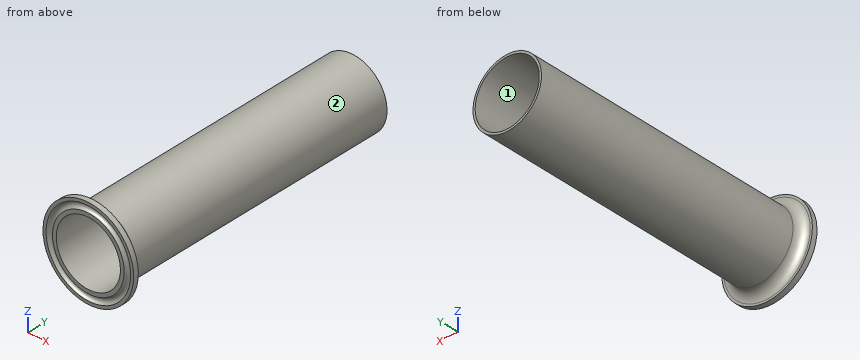
from build123d import *

# Parameters (mm, degrees)
SKETCH_1_R          = 25.25
EXTRUDE_1_DEPTH     = 2.8
SKETCH_2_R          = 19.05
EXTRUDE_2_DEPTH     = 157.2
FILLET_1_R          = 5
SKETCH_3_R          = 17.85
CUT_EXTRUDE_1_DEPTH = 164.936344354
SKETCH_5_R          = 1.8


with BuildPart() as part:
    # 스케치1 → 보스-돌출1 (new body)
    with BuildSketch(Plane(origin=(0, 0, 0), x_dir=(1, 0, 0), z_dir=(0, 1, 0))):
        with Locations(Location((0, 0, 0), (0, 0, 270))):
            Circle(SKETCH_1_R)
    extrude(amount=EXTRUDE_1_DEPTH)

    # 스케치2 → 보스-돌출2 (add)
    with BuildSketch(Plane(origin=(0, 2.8, 0), x_dir=(1, 0, 0), z_dir=(0, 1, 0))):
        with Locations(Location((0, 0, 0), (0, 0, 270))):
            Circle(SKETCH_2_R)
    extrude(amount=EXTRUDE_2_DEPTH)

    # 필렛1
    fillet_1_edges = [part.edges().sort_by_distance(p)[0] for p in [
        (0, 2.8, -19.05),
    ]]
    fillet(fillet_1_edges, radius=FILLET_1_R)

    # 스케치3 → 컷-돌출1 (cut, through all)
    with BuildSketch(Plane(origin=(0, 160, 0), x_dir=(1, 0, 0), z_dir=(0, 1, 0))):
        with Locations(Location((0, 0, 0), (0, 0, 270))):
            Circle(SKETCH_3_R)
    extrude(amount=-CUT_EXTRUDE_1_DEPTH, mode=Mode.SUBTRACT)

    # 컷-스윕1: sweep along a path in 스케치4
    with BuildLine(Plane.XZ) as sweep_1_path:
        CenterArc((0, 0), 21.75, 0, 360)
    # 스케치5 → 컷-스윕1 (sweep, cut)
    with BuildSketch(Plane.XY):
        with Locations((-21.75, 0)):
            Circle(SKETCH_5_R)
    sweep(path=sweep_1_path.line, mode=Mode.SUBTRACT)


solid = part.part
CAD build for the part. Positions are in the model's coordinates, mm. Face numbers are marked on the shaded views. Coordinates: 2 decimals unless noted, no trailing zeros. Loops run counter-clockwise (first coordinate to the right, second up) from the corner with the lowest first, then second, coordinate; pieces in that order, holes last. Notation, with made-up numbers: (28.5, -20) - (52.5, -20) arc R14 cw to (52.5, -6) - close; hole circle Ø4 at (18, 41). An arc over 180 degrees is marked (long way). Use one line per item in the form item = value. Start each with the question number.
1) Drill centre lines: L1, parallel to X at y = 73, z = 0; L2, parallel to Y at x = 19, z = -14; L3, parallel to X at y = 128, z = -7.5. Where is each one in solid material? Low to high. Write a range as from..to.
2) Flat gauge pins, fed straight in: pin 1 (1 mm diameter, centred on x = -10.5, y = 119, fed in from -Z); pin 2 (1.5 mm diameter, centred on x = -16, y = 16.5, fed in from +Z); pin 3 (5 mm diameter, centred on x = -17.5, y = 79.5, fed in from +Z). Where does each tip first touch, or does it go through?
3) Band-saw the part on B-B (z = 0). Give the cut face in (x, y), and give its area (3 significant figures).
4) Band-saw the part on C-C (y = 132.5). Give the cut face in (x, z).
5) Band-saw the part on A-A (x = 0). Give the cut face in (y, z).
6) Two-plate mould, pull along X, no slides. Class the marked faces 1 and 2: +X half, -X half, draft (parallel to the pull), parting line (faces both ways), or undercut.
Check values:
q1.L1 = -19.05..-17.85, 17.85..19.05
q1.L2 = 0..2.82
q1.L3 = -17.51..-16.2, 16.2..17.51
q2.pin_1 = -16.21
q2.pin_2 = 11.42
q2.pin_3 = 11.74
q3.outline = (-25.25, 0) - (-23.55, 0) arc R1.8 cw to (-19.95, 0) - (-17.85, 0) - (-17.85, 160) - (-19.05, 160) - (-19.05, 7.8) arc R5 cw to (-24.05, 2.8) - (-25.25, 2.8) - close; (17.85, 0) - (19.95, 0) arc R1.8 cw to (23.55, 0) - (25.25, 0) - (25.25, 2.8) - (24.05, 2.8) arc R5 cw to (19.05, 7.8) - (19.05, 160) - (17.85, 160) - close
q3.area = 419 mm2
q4.outline = circle Ø38.1 at (0, 0); hole circle Ø35.7 at (0, 0)
q5.outline = (0, -25.25) - (2.8, -25.25) - (2.8, -24.05) arc R5 cw to (7.8, -19.05) - (160, -19.05) - (160, -17.85) - (0, -17.85) - (0, -19.95) arc R1.8 cw to (0, -23.55) - close; (0, 17.85) - (160, 17.85) - (160, 19.05) - (7.8, 19.05) arc R5 cw to (2.8, 24.05) - (2.8, 25.25) - (0, 25.25) - (0, 23.55) arc R1.8 cw to (0, 19.95) - close
q6.face_1 = undercut
q6.face_2 = parting line
